The listing builds one solid part. Answer for the finished solid, in the listing's coordinates (mm). A direction names the side the tool comes from. Give positions to 0.01 mm unless a question says otherwise; leave off trailing zeros. Loops run counter-clockwise (first coordinate to the right, second up) from the corner with the lowest first, then second, coordinate; pieces in that order, holes last. Notation, with made-up numbers: M 7,84.5 L 42,84.5 A16 cw 42,88.5 Z; hole C -21,5.25 d11. An arc over 180 degrees is marked long. Use one line per item in the form item = value. Start each with the question number.
1. The part is cut by section A-A (z = -5). Write down the section's boundary in (x, y).
2. The part is cut by section D-D (z = -29). Write down the section's boundary in (x, y) (3 decimals).
3. Each of these flat-tipped pins is pushed along its axis until it touches: pin 1 Ø7 at (y, z) = (-10.5, -4.5) entering from -X; pin 2 Ø4.5 at (x, y) = (-52, -11.5) entering from +Z; pin 3 Ø4 at (y, z) = (-2.5, -26.5) entering from -X; pin 4 Ø2.5 at (y, z) = (8, -4) entering from +X. Where does it stop, or does it pass through?
4. The mould has two halves that part along Y. Classify faces 1 (the face through (51.836, -6.245, -22.058)), 2 (the face through (42, -9, -4)): released by +Y, released by -Y, zero draft, split by the parting line, or undercut.
5. Straight lines are drawn through the part: line 1 (Y direction, x = 35, z = -25); line 2 (Z direction, x = -44.5, y = -12.25); line 3 (X direction, y = -12, z = -7.5). For each, find the intervals that lie inside material, in ascending order. Write a range as from..to.
6. The part is cut by section B-B (x = -26.5). Write down the section's boundary in (y, z), and give its area (3 significant figures).
7. The part is cut by section C-C (y = 10). Write down the section's boundary in (x, z), and give its area (3 significant figures).
8. For faces 3 (the face through (42, 9, -4)), 4 (the face through (-42, -9, -4)), 5 (the face through (1, 4.8, -16)), 6 (the face through (-51.836, 6.245, -22.058)), determine the directions among +Z, -Z, +X, -X, +Y, -Y from which every point of the face is accessible in a straight line to the end or side of a thin tool.
Solid Edge part; units mm, degrees
sketch "Sketch1" plane through (0, 0, 0) normal (0, 0, 1) x (1, 0, 0)
  line L0 (-60.5, -14) -> (60.5, -14)
  line L1 (60.5, -14) -> (60.5, 14)
  line L2 (60.5, 14) -> (-60.5, 14)
  line L3 (-60.5, 14) -> (-60.5, -14)
extrude "Protrusion1" add sketch "Sketch1" against normal blind 40
sketch "Sketch2" plane through (0, -14, -20) normal (0, -1, 0) x (1, 0, 0)
  line L0 (60.5, 20) -> (42, 20)
  line L1 (42, 20) -> (42, 11.5)
  line L2 (42, 11.5) -> (60.5, 11.5)
  line L3 (60.5, 11.5) -> (60.5, 20)
extrude "ExtrudedCutout_11" cut sketch "Sketch2" against normal blind 28
sketch "Sketch3" plane through (0, -14, -20) normal (0, -1, 0) x (1, 0, 0)
  line L0 (-60.5, 11.5) -> (-42, 11.5)
  line L1 (-42, 11.5) -> (-42, 20)
  line L2 (-42, 20) -> (-60.5, 20)
  line L3 (-60.5, 20) -> (-60.5, 11.5)
extrude "ExtrudedCutout_12" cut sketch "Sketch3" against normal blind 28
sketch "Sketch4" plane through (0, 9.325, 0) normal (0, 0, 1) x (1, 0, 0)
  line L0 (60.5, -4.675) -> (60.5, -1.675)
  line L1 (60.5, -1.675) -> (42, -4.675)
  line L2 (42, -4.675) -> (60.5, -4.675)
extrude "ExtrudedCutout_23" cut sketch "Sketch4" against normal blind 33
sketch "Sketch5" plane through (0, -9.325, 0) normal (0, 0, 1) x (1, 0, 0)
  line L0 (60.5, 4.675) -> (60.5, 1.675)
  line L1 (60.5, 1.675) -> (42, 4.675)
  line L2 (42, 4.675) -> (60.5, 4.675)
  line L3 (-60.5, 13.975) -> (-60.5, 16.975)
  line L4 (-60.5, 16.975) -> (-42, 13.975)
  line L5 (-42, 13.975) -> (-60.5, 13.975)
extrude "ExtrudedCutout_24" cut sketch "Sketch5" against normal blind 33
sketch "Sketch6" plane through (0, -9.325, 0) normal (0, 0, 1) x (1, 0, 0)
  line L0 (-60.5, 4.675) -> (-60.5, 1.675)
  line L1 (-60.5, 1.675) -> (-42, 4.675)
  line L2 (-42, 4.675) -> (-60.5, 4.675)
extrude "ExtrudedCutout_26" cut sketch "Sketch6" against normal blind 33
sketch "Sketch7" plane through (0, 0, 0) normal (0, 0, 1) x (0, 1, 0)
  line L0 (-4.8, -60.5) -> (4.8, -60.5)
  line L1 (4.8, -60.5) -> (4.8, 60.5)
  line L2 (4.8, 60.5) -> (-4.8, 60.5)
  line L3 (-4.8, 60.5) -> (-4.8, -60.5)
extrude "ExtrudedCutout_27" cut sketch "Sketch7" against normal blind 33
chamfer "Chamfer_7" distance 3 distance2 18 1 edges at (60.5, 0, -33) measured on face at (60.5, -9.6133, -34.435)
chamfer "Chamfer_8" distance 3 distance2 18 1 edges at (-60.5, 0, -33) measured on face at (-60.5, 9.6133, -34.435)
Derived:
q1.outline = M -42,-14 L 42,-14 L 42,-4.8 L -42,-4.8 Z; M -42,4.8 L 42,4.8 L 42,14 L -42,14 Z
q2.outline = M -60.5,-14 L 60.5,-14 L 60.5,-7.65 L 42.925,-4.8 L -42.925,-4.8 L -60.5,-7.65 Z; M -60.5,7.65 L -42.925,4.8 L 42.925,4.8 L 60.5,7.65 L 60.5,14 L -60.5,14 Z
q3.pin_1 = -42
q3.pin_2 = -8.5
q3.pin_3 = through
q3.pin_4 = 42
q4.face_1 = undercut
q4.face_2 = zero draft
q5.line_1 = -14..-4.8, 4.8..14
q5.line_2 = -40..-8.5
q5.line_3 = -42..42
q6.outline = M -14,-40 L 14,-40 L 14,0 L 4.8,0 L 4.8,-33 L -4.8,-33 L -4.8,0 L -14,0 Z
q6.area = 803 mm2
q7.outline = M -60.5,-40 L 60.5,-40 L 60.5,-8.5 L 42,-8.5 L 42,0 L -42,0 L -42,-8.5 L -60.5,-8.5 Z
q7.area = 4,530 mm2
q8.face_3 = +Z, +X, +Y, -Y
q8.face_4 = +Z, -X, +Y, -Y
q8.face_5 = +Z, +X, -X
q8.face_6 = +Z, -X
